from build123d import *

# Parameters (mm, degrees)
F1_DEPTH      = 7
F5_DEPTH      = 0.8
F6_REACH      = 40.8395042988
F7_W          = 36.7298226772
F7_H          = 7
F8_DEPTH      = 1
F9_DEPTH      = 45
F10_T1_DEPTH  = 7
F10_T3_DEPTH  = 21.8461795352
F10_T5_DEPTH  = 11.8964874596
F10_T7_DEPTH  = 11.956767541
F10_T12_DEPTH = 5.3023503656


# Not quite as in the source:
# - a fillet or chamfer that OpenCascade refuses, or shapes differently, is made with other operations: its cross-section is extruded or revolved along the edge and cut away or added


with BuildPart() as f1:
    # F0 (on Top) → F1 (new body)
    with BuildSketch(Plane.XY):
        with BuildLine():
            Line((0, 0), (0, -36.7298226772))
            Line((0, -36.7298226772), (24, -18.0982437298))
            Line((24, -18.0982437298), (24, -10))
            Line((24, -10), (59, -10))
            ThreePointArc((59, -10), (65.3245553203, -7.7459666924), (68.7979589711, -2))
            ThreePointArc((68.7979589711, -2), (68.9493615301, -1.0050896201), (69, 0))
            Line((69, 0), (0, 0))
        make_face()
        Polygon((33.4652661258, -8), (28.0146803707, -8), (28.0146803707, -3.3182508079), align=None, mode=Mode.SUBTRACT)
        Polygon((41, -3.4142135624), (45.5857864376, -8), (36.4142135624, -8), align=None, mode=Mode.SUBTRACT)
        Polygon((29.5494142449, -2), (39.5857864376, -2), (34.9483778196, -6.637408618), align=None, mode=Mode.SUBTRACT)
        Polygon((42.4142135624, -2), (51.5857864376, -2), (47, -6.5857864376), align=None, mode=Mode.SUBTRACT)
        Polygon((53, -3.4142135624), (57.5857864376, -8), (48.4142135624, -8), align=None, mode=Mode.SUBTRACT)
        with BuildLine():
            ThreePointArc((66.7459666924, -2), (64.4007894962, -5.9018194498), (60.3067648391, -7.8925512767))
            Line((60.3067648391, -7.8925512767), (54.4142135624, -2))
            Line((54.4142135624, -2), (66.7459666924, -2))
        make_face(mode=Mode.SUBTRACT)
    extrude(amount=F1_DEPTH)

    # F4 (on face) → F5 (cut)
    with BuildSketch(Plane(origin=(0, 0, 0), x_dir=(0.9781476007, 0, 0.2079116908), z_dir=(0.2079116908, 0, -0.9781476007))):
        Polygon((19, 15.5), (0, 30.75), (0, 28.1854591432), (17, 14.5407223011), (17, 5.1), (19, 5.1), align=None)
        with BuildLine():
            Line((17, 14.5407223011), (0, 28.1854591432))
            Line((0, 28.1854591432), (0, 0))
            Line((0, 0), (19, 0))
            Line((19, 0), (19, 1.9))
            Line((19, 1.9), (16, 1.9))
            ThreePointArc((16, 1.9), (14.4, 3.5), (16, 5.1))
            Line((16, 5.1), (17, 5.1))
            Line((17, 5.1), (17, 14.5407223011))
        make_face()
    extrude(amount=-F5_DEPTH, mode=Mode.SUBTRACT)

    f6_end = Plane(origin=(20.8323918984, -11.3984937311, 7), x_dir=(1, 0, 0), z_dir=(0, 0, 1))
    # F4 (on face) → F6 (cut, up to a plane its end follows)
    with BuildSketch(Plane(origin=(0, 0, 0), x_dir=(0.9781476007, 0, 0.2079116908), z_dir=(0.2079116908, 0, -0.9781476007))):
        with BuildLine():
            Line((17, 14.5407223011), (0, 28.1854591432))
            Line((0, 28.1854591432), (0, 0))
            Line((0, 0), (19, 0))
            Line((19, 0), (19, 1.9))
            Line((19, 1.9), (16, 1.9))
            ThreePointArc((16, 1.9), (14.4, 3.5), (16, 5.1))
            Line((16, 5.1), (17, 5.1))
            Line((17, 5.1), (17, 14.5407223011))
        make_face()
    f6_long = extrude(amount=-F6_REACH, mode=Mode.PRIVATE)
    add(split(f6_long, bisect_by=f6_end, keep=Keep.BOTTOM, mode=Mode.PRIVATE), mode=Mode.SUBTRACT)

    # F7 (on face) → F8 (cut)
    with BuildSketch(Plane(origin=(0, 0, 0), x_dir=(0, -1, 0), z_dir=(-1, 0, 0))):
        with Locations((18.3649113386, 3.5)):
            Rectangle(F7_W, F7_H)
    extrude(amount=-F8_DEPTH, mode=Mode.SUBTRACT)

    # F2 (on face) → F9 (cut)
    with BuildSketch(Plane(origin=(0, 0, 0), x_dir=(-1, 0, 0), z_dir=(0, 1, 0))):
        Polygon((0, 4), (-6.7871916141, 4), (0, 0.9781476007), align=None)
        Polygon((-13.5253019358, 7), (-6.7871916141, 4), (0, 4), (0, 7), align=None)
    extrude(amount=-F9_DEPTH, mode=Mode.SUBTRACT)

    # F10: fillet of radius 2 on 5 edges, made by hand

    # F10_s2 → F10_t1 (join)
    with BuildSketch(Plane.XY):
        with BuildLine():
            ThreePointArc((24, -12), (24.5857864376, -10.5857864376), (26, -10))
            Line((26, -10), (24, -10))
            Line((24, -10), (24, -12))
        make_face()
    extrude(amount=F10_T1_DEPTH)

    # F10_s4 → F10_t3 (cut)
    with BuildSketch(Plane.XY.offset(-10.2114016246)):
        with BuildLine():
            ThreePointArc((4.2264416068, -33.4487693246), (2.1204783157, -33.6651760692), (1, -31.8689462379))
            Line((1, -31.8689462379), (1, -35.9535068877))
            Line((1, -35.9535068877), (4.2264416068, -33.4487693246))
        make_face()
    extrude(amount=F10_T3_DEPTH, mode=Mode.SUBTRACT)

    # F10_s6 → F10_t5 (cut)
    with BuildSketch(Plane.XY.offset(-2.4482437298)):
        with BuildLine():
            ThreePointArc((24, -17.1189462379), (23.7962298313, -17.9984679222), (23.2264416068, -18.6987693246))
            Line((23.2264416068, -18.6987693246), (24, -18.0982437298))
            Line((24, -18.0982437298), (24, -17.1189462379))
        make_face()
    extrude(amount=F10_T5_DEPTH, mode=Mode.SUBTRACT)

    # F10_s8 → F10_t7 (cut)
    with BuildSketch(Plane.XZ.offset(15.3359324944)):
        with BuildLine():
            ThreePointArc((13.9504150591, 7), (13.5345916775, 6.9562952015), (13.136941773, 6.8270909153))
            Line((13.136941773, 6.8270909153), (13.5253019358, 7))
            Line((13.5253019358, 7), (13.9504150591, 7))
        make_face()
    extrude(amount=F10_T7_DEPTH, mode=Mode.SUBTRACT)


with BuildPart() as f10_tool10:
    # F10_s11 → F10_t12 (new body)
    with BuildSketch(Plane(origin=(0, -0.1012401159, -0.6066769302), x_dir=(1, 0, 0), z_dir=(0, -0.1646003505, -0.9863603422))):
        with BuildLine():
            ThreePointArc((1, 28.0074292273), (1.2043011265, 27.126824006), (1.7754655557, 26.4261274235))
            Line((1.7754655557, 26.4261274235), (1, 27.0266353601))
            Line((1, 27.0266353601), (1, 28.0074292273))
        make_face()
    extrude(amount=F10_T12_DEPTH)

    split(bisect_by=Plane(origin=(-0.1663293527, 0, 0.7825180806), x_dir=(0, 1, 0), z_dir=(-0.2079116908, 0, 0.9781476007)), keep=Keep.TOP)


with BuildPart() as f1_1:
    add(f1.part)

    # F10_t9: cut F10_tool10
    add(f10_tool10.part, mode=Mode.SUBTRACT)

    # F11: F1 across plane


with BuildPart() as f1_2:
    add(f1_1.part)
    add(f1_1.part.mirror(Plane.XZ))


solid = f1_2.part
Verification items for the finished model (mm, model axes). A direction names the side the tool comes from. Coordinates: 2 decimals unless noted, no trailing zeros. Order: outer loops, then holes, each group sorted by start corner. A loop starts at its lowest first (then second) coordinate and runs counter-clockwise, first axis right, second up. Notation, with made-up numbers: (44.25, 37.25) -> (97.25, 37.25) arc R25 ccw to (97.25, 53.25) -> close; hole circle Ø8 at (74, 42.5). An arc over 180 degrees is marked (long way). Use CSV: the item, a comma, the result in double quotes. Start each with the question number.
Q1. Section check D-D, the plane y = -11. Record the cut outline in (x, z), and give its area (3 significant figures).
Q2. Section check B-B, the plane y = 20. Record the cut outline in (x, z).
Q3. Section check C-C, the plane x = 10.5. Record the cut outline in (y, z).
Q4. Depth check by flat-ended pin: P1, Ø4, axis at y = -3.5, z = 1.5, coming from the +X side; P2, Ø4, axis at x = 17.5, z = 6, coming from the +Y side; P3, Ø4, axis at x = 17, z = 4.5, coming from the +Y side. Enter the tip coordinate at first touch or a pass-through.
Q5. Thickness scan on line 1 along Y through (x, z) = (31, 6.25); line 2 along Y through (x, z) = (40, 5.5); line 3 along Y through (x, z) = (36, 6.5). Record the ranges inside material, lowest first.
Q6. Section check A-A, the plane x = 64. Record the cut outline in (y, z) (3 decimals), and give its area (3 significant figures).
Q7. Draft check along Y on faces 6 (the flat face through (47, -2, 3)), 7 (the cylindrical face through (23.8, -17.99, 3.45)), 8 (the flat face through (15.7, 24.54, 3.45)). Enter one of: +Y half, -Y half, draft (parallel to the pull), parting line (faces both ways), or undercut.
Q8. Tool access check on faces 1 (the cylindrical face through (13.672, 3.465, 4.94)), 2 (the flat face through (24, -15, 3)), 3 (the flat face through (27, 0, 0)), 4 (the flat face through (12.25, -18.42, 3.42)), 5 (the flat face through (38.675, -5.739, 3.451)). Record the directions out of +Z, -Z, +X, -X, +Y, -Y that give a thin tool (end or side, any length) a straight path to the whole face; none if there is none.
Returned:
1,outline,"(1, 0) -> (24.27, 0) -> (24.27, 7) -> (15.89, 7) -> (16.46, 4.32) -> (18.42, 4.73) -> (18.58, 3.95) -> (1, 0.21) -> close"
1,area,"82.4 mm^2"
2,outline,"(1, 0) -> (21.55, 0) -> (21.55, 7) -> (13.95, 7) arc R2 ccw to (13.14, 6.83) -> (9.33, 5.13) -> (9.81, 2.9) -> (12.93, 3.57) -> (13.1, 2.78) -> (1, 0.21) -> close"
3,outline,"(-28.58, 0) -> (28.58, 0) -> (28.58, 5.65) -> (19, 5.65) -> (19.43, 3.05) -> (22, 3.05) -> (22.13, 2.23) -> (-22.13, 2.23) -> (-22, 3.05) -> (-19.43, 3.05) -> (-19, 5.65) -> (-28.58, 5.65) -> close"
4,P1,"stops at x = 68.89"
4,P2,"stops at y = 24.7"
4,P3,"stops at y = 25.09"
5,line 1,"y = -10 to -8, -5.88 to -3.25, -2 to 2, 3.25 to 5.88, 8 to 10"
5,line 2,"y = -10 to -8, -4.41 to 4.41, 8 to 10"
5,line 3,"y = -10 to -5.59, -2 to 2, 5.59 to 10"
6,outline,"(-8.66, 0) -> (-6.245, 0) -> (-6.245, 7) -> (-8.66, 7) -> close; (-2, 0) -> (2, 0) -> (2, 7) -> (-2, 7) -> close; (6.245, 0) -> (8.66, 0) -> (8.66, 7) -> (6.245, 7) -> close"
6,area,"61.8 mm^2"
7,face 6,"undercut"
7,face 7,"-Y half"
7,face 8,"+Y half"
8,face 1,"-X"
8,face 2,"+Z, -Z, +X, -Y"
8,face 3,"-Z, +X, -X, +Y, -Y"
8,face 4,"none"
8,face 5,"+Z, -Z"
